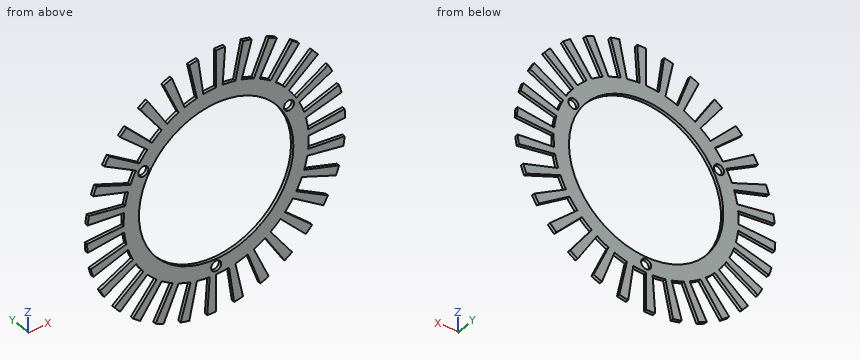
from build123d import *

# Parameters (mm, degrees)
SKETCH1_R           = 30.25
SKETCH1_R_2         = 25.25
EXTRUDE_THIN1_DEPTH = 1
SKETCH2_R           = 1.65
CUT_EXTRUDE3_DEPTH  = 10
BOSS_EXTRUDE1_DEPTH = 1


with BuildPart() as part:
    # Sketch1 → Extrude-Thin1 (new body)
    with BuildSketch(Plane(origin=(0, 0, 0), x_dir=(1, 0, 0), z_dir=(0, 1, 0))):
        Circle(SKETCH1_R)
        Circle(SKETCH1_R_2, mode=Mode.SUBTRACT)
    extrude(amount=-EXTRUDE_THIN1_DEPTH)

    # Sketch2 → Cut-Extrude3 (cut)
    with BuildSketch(Plane(origin=(0, 0, 0), x_dir=(1, 0, 0), z_dir=(0, 1, 0))):
        with Locations((0, 27.5)):
            Circle(SKETCH2_R)
        with Locations((23.815698604, -13.75)):
            Circle(SKETCH2_R)
        with Locations((-23.815698604, -13.75)):
            Circle(SKETCH2_R)
    extrude(amount=-CUT_EXTRUDE3_DEPTH, mode=Mode.SUBTRACT)

    # Sketch5 → Boss-Extrude1 (add)
    with BuildSketch(Plane.XZ.offset(1)):
        with BuildLine():
            Line((0, 42.25), (0, 30.25))
            ThreePointArc((0, 30.25), (1.055709775, 30.231572517), (2.110133331, 30.17631252))
            Line((2.110133331, 30.17631252), (2.947211016, 42.147081123))
            ThreePointArc((2.947211016, 42.147081123), (1.474503736, 42.224262442), (0, 42.25))
        make_face()
        with BuildLine():
            Line((8.784268937, 41.326736131), (6.289328647, 29.588964922))
            ThreePointArc((6.289328647, 29.588964922), (7.318137342, 29.35144572), (8.338030013, 29.078166302))
            Line((8.338030013, 29.078166302), (11.645678283, 40.613306653))
            ThreePointArc((11.645678283, 40.613306653), (10.221200089, 40.994994435), (8.784268937, 41.326736131))
        make_face()
        with BuildLine():
            Line((17.18462317, 38.597295585), (12.303783453, 27.634750094))
            ThreePointArc((12.303783453, 27.634750094), (13.26072719, 27.188519901), (14.201514774, 26.709164684))
            Line((14.201514774, 26.709164684), (19.835173528, 37.304535798))
            ThreePointArc((19.835173528, 37.304535798), (18.521180952, 37.974048456), (17.18462317, 38.597295585))
        make_face()
        with BuildLine():
            Line((24.833926909, 34.180968012), (17.780503882, 24.47276408))
            ThreePointArc((17.780503882, 24.47276408), (18.623759629, 23.837325297), (19.444325193, 23.172844404))
            Line((19.444325193, 23.172844404), (27.157776509, 32.365377722))
            ThreePointArc((27.157776509, 32.365377722), (26.011697333, 33.29345434), (24.833926909, 34.180968012))
        make_face()
        with BuildLine():
            Line((31.397868876, 28.270768119), (22.480130971, 20.241200842))
            ThreePointArc((22.480130971, 20.241200842), (23.172844404, 19.444325193), (23.837325297, 18.623759629))
            Line((23.837325297, 18.623759629), (33.29345434, 26.011697333))
            ThreePointArc((33.29345434, 26.011697333), (32.365377722, 27.157776509), (31.397868876, 28.270768119))
        make_face()
        with BuildLine():
            Line((36.58957331, 21.125), (26.197268464, 15.125))
            ThreePointArc((26.197268464, 15.125), (26.709164684, 14.201514774), (27.188519901, 13.26072719))
            Line((27.188519901, 13.26072719), (37.974048456, 18.521180952))
            ThreePointArc((37.974048456, 18.521180952), (37.304535798, 19.835173528), (36.58957331, 21.125))
        make_face()
        with BuildLine():
            Line((40.182137813, 13.055968012), (28.769459618, 9.34776408))
            ThreePointArc((28.769459618, 9.34776408), (29.078166302, 8.338030013), (29.35144572, 7.318137342))
            Line((29.35144572, 7.318137342), (40.994994435, 10.221200089))
            ThreePointArc((40.994994435, 10.221200089), (40.613306653, 11.645678283), (40.182137813, 13.055968012))
        make_face()
        with BuildLine():
            Line((42.018550079, 4.416327573), (30.084287335, 3.161986014))
            ThreePointArc((30.084287335, 3.161986014), (30.17631252, 2.110133331), (30.231572517, 1.055709775))
            Line((30.231572517, 1.055709775), (42.224262442, 1.474503736))
            ThreePointArc((42.224262442, 1.474503736), (42.147081123, 2.947211016), (42.018550079, 4.416327573))
        make_face()
        with BuildLine():
            Line((42.018550079, -4.416327573), (30.084287335, -3.161986014))
            ThreePointArc((30.084287335, -3.161986014), (29.955609079, -4.209986304), (29.790434529, -5.252857374))
            Line((29.790434529, -5.252857374), (41.608127565, -7.336635506))
            ThreePointArc((41.608127565, -7.336635506), (41.838825904, -5.880063516), (42.018550079, -4.416327573))
        make_face()
        with BuildLine():
            Line((40.182137813, -13.055968012), (28.769459618, -9.34776408))
            ThreePointArc((28.769459618, -9.34776408), (28.425701779, -10.346109336), (28.047311601, -11.331849451))
            Line((28.047311601, -11.331849451), (39.173517855, -15.827128572))
            ThreePointArc((39.173517855, -15.827128572), (39.702013228, -14.450351056), (40.182137813, -13.055968012))
        make_face()
        with BuildLine():
            Line((36.58957331, -21.125), (26.197268464, -15.125))
            ThreePointArc((26.197268464, -15.125), (25.653454909, -16.030057743), (25.07838657, -16.91558533))
            Line((25.07838657, -16.91558533), (35.02683744, -23.625900172))
            ThreePointArc((35.02683744, -23.625900172), (35.830032063, -22.389088914), (36.58957331, -21.125))
        make_face()
        with BuildLine():
            Line((31.397868876, -28.270768119), (22.480130971, -20.241200842))
            ThreePointArc((22.480130971, -20.241200842), (21.76002896, -21.013415706), (21.013415706, -21.76002896))
            Line((21.013415706, -21.76002896), (29.349316152, -30.392106564))
            ThreePointArc((29.349316152, -30.392106564), (30.392106564, -29.349316152), (31.397868876, -28.270768119))
        make_face()
        with BuildLine():
            Line((24.833926909, -34.180968012), (17.780503882, -24.47276408))
            ThreePointArc((17.780503882, -24.47276408), (16.91558533, -25.07838657), (16.030057743, -25.653454909))
            Line((16.030057743, -25.653454909), (22.389088914, -35.830032063))
            ThreePointArc((22.389088914, -35.830032063), (23.625900172, -35.02683744), (24.833926909, -34.180968012))
        make_face()
        with BuildLine():
            Line((17.18462317, -38.597295585), (12.303783453, -27.634750094))
            ThreePointArc((12.303783453, -27.634750094), (11.331849451, -28.047311601), (10.346109336, -28.425701779))
            Line((10.346109336, -28.425701779), (14.450351056, -39.702013228))
            ThreePointArc((14.450351056, -39.702013228), (15.827128572, -39.173517855), (17.18462317, -38.597295585))
        make_face()
        with BuildLine():
            Line((8.784268937, -41.326736131), (6.289328647, -29.588964922))
            ThreePointArc((6.289328647, -29.588964922), (5.252857374, -29.790434529), (4.209986304, -29.955609079))
            Line((4.209986304, -29.955609079), (5.880063516, -41.838825904))
            ThreePointArc((5.880063516, -41.838825904), (7.336635506, -41.608127565), (8.784268937, -41.326736131))
        make_face()
        with BuildLine():
            Line((0, -42.25), (0, -30.25))
            ThreePointArc((0, -30.25), (-1.055709775, -30.231572517), (-2.110133331, -30.17631252))
            Line((-2.110133331, -30.17631252), (-2.947211016, -42.147081123))
            ThreePointArc((-2.947211016, -42.147081123), (-1.474503736, -42.224262442), (0, -42.25))
        make_face()
        with BuildLine():
            Line((-8.784268937, -41.326736131), (-6.289328647, -29.588964922))
            ThreePointArc((-6.289328647, -29.588964922), (-7.318137342, -29.35144572), (-8.338030013, -29.078166302))
            Line((-8.338030013, -29.078166302), (-11.645678283, -40.613306653))
            ThreePointArc((-11.645678283, -40.613306653), (-10.221200089, -40.994994435), (-8.784268937, -41.326736131))
        make_face()
        with BuildLine():
            Line((-17.18462317, -38.597295585), (-12.303783453, -27.634750094))
            ThreePointArc((-12.303783453, -27.634750094), (-13.26072719, -27.188519901), (-14.201514774, -26.709164684))
            Line((-14.201514774, -26.709164684), (-19.835173528, -37.304535798))
            ThreePointArc((-19.835173528, -37.304535798), (-18.521180952, -37.974048456), (-17.18462317, -38.597295585))
        make_face()
        with BuildLine():
            Line((-24.833926909, -34.180968012), (-17.780503882, -24.47276408))
            ThreePointArc((-17.780503882, -24.47276408), (-18.623759629, -23.837325297), (-19.444325193, -23.172844404))
            Line((-19.444325193, -23.172844404), (-27.157776509, -32.365377722))
            ThreePointArc((-27.157776509, -32.365377722), (-26.011697333, -33.29345434), (-24.833926909, -34.180968012))
        make_face()
        with BuildLine():
            Line((-31.397868876, -28.270768119), (-22.480130971, -20.241200842))
            ThreePointArc((-22.480130971, -20.241200842), (-23.172844404, -19.444325193), (-23.837325297, -18.623759629))
            Line((-23.837325297, -18.623759629), (-33.29345434, -26.011697333))
            ThreePointArc((-33.29345434, -26.011697333), (-32.365377722, -27.157776509), (-31.397868876, -28.270768119))
        make_face()
        with BuildLine():
            Line((-36.58957331, -21.125), (-26.197268464, -15.125))
            ThreePointArc((-26.197268464, -15.125), (-26.709164684, -14.201514774), (-27.188519901, -13.26072719))
            Line((-27.188519901, -13.26072719), (-37.974048456, -18.521180952))
            ThreePointArc((-37.974048456, -18.521180952), (-37.304535798, -19.835173528), (-36.58957331, -21.125))
        make_face()
        with BuildLine():
            Line((-40.182137813, -13.055968012), (-28.769459618, -9.34776408))
            ThreePointArc((-28.769459618, -9.34776408), (-29.078166302, -8.338030013), (-29.35144572, -7.318137342))
            Line((-29.35144572, -7.318137342), (-40.994994435, -10.221200089))
            ThreePointArc((-40.994994435, -10.221200089), (-40.613306653, -11.645678283), (-40.182137813, -13.055968012))
        make_face()
        with BuildLine():
            Line((-42.018550079, -4.416327573), (-30.084287335, -3.161986014))
            ThreePointArc((-30.084287335, -3.161986014), (-30.17631252, -2.110133331), (-30.231572517, -1.055709775))
            Line((-30.231572517, -1.055709775), (-42.224262442, -1.474503736))
            ThreePointArc((-42.224262442, -1.474503736), (-42.147081123, -2.947211016), (-42.018550079, -4.416327573))
        make_face()
        with BuildLine():
            Line((-42.018550079, 4.416327573), (-30.084287335, 3.161986014))
            ThreePointArc((-30.084287335, 3.161986014), (-29.955609079, 4.209986304), (-29.790434529, 5.252857374))
            Line((-29.790434529, 5.252857374), (-41.608127565, 7.336635506))
            ThreePointArc((-41.608127565, 7.336635506), (-41.838825904, 5.880063516), (-42.018550079, 4.416327573))
        make_face()
        with BuildLine():
            Line((-40.182137813, 13.055968012), (-28.769459618, 9.34776408))
            ThreePointArc((-28.769459618, 9.34776408), (-28.425701779, 10.346109336), (-28.047311601, 11.331849451))
            Line((-28.047311601, 11.331849451), (-39.173517855, 15.827128572))
            ThreePointArc((-39.173517855, 15.827128572), (-39.702013228, 14.450351056), (-40.182137813, 13.055968012))
        make_face()
        with BuildLine():
            Line((-36.58957331, 21.125), (-26.197268464, 15.125))
            ThreePointArc((-26.197268464, 15.125), (-25.653454909, 16.030057743), (-25.07838657, 16.91558533))
            Line((-25.07838657, 16.91558533), (-35.02683744, 23.625900172))
            ThreePointArc((-35.02683744, 23.625900172), (-35.830032063, 22.389088914), (-36.58957331, 21.125))
        make_face()
        with BuildLine():
            Line((-31.397868876, 28.270768119), (-22.480130971, 20.241200842))
            ThreePointArc((-22.480130971, 20.241200842), (-21.76002896, 21.013415706), (-21.013415706, 21.76002896))
            Line((-21.013415706, 21.76002896), (-29.349316152, 30.392106564))
            ThreePointArc((-29.349316152, 30.392106564), (-30.392106564, 29.349316152), (-31.397868876, 28.270768119))
        make_face()
        with BuildLine():
            Line((-24.833926909, 34.180968012), (-17.780503882, 24.47276408))
            ThreePointArc((-17.780503882, 24.47276408), (-16.91558533, 25.07838657), (-16.030057743, 25.653454909))
            Line((-16.030057743, 25.653454909), (-22.389088914, 35.830032063))
            ThreePointArc((-22.389088914, 35.830032063), (-23.625900172, 35.02683744), (-24.833926909, 34.180968012))
        make_face()
        with BuildLine():
            Line((-17.18462317, 38.597295585), (-12.303783453, 27.634750094))
            ThreePointArc((-12.303783453, 27.634750094), (-11.331849451, 28.047311601), (-10.346109336, 28.425701779))
            Line((-10.346109336, 28.425701779), (-14.450351056, 39.702013228))
            ThreePointArc((-14.450351056, 39.702013228), (-15.827128572, 39.173517855), (-17.18462317, 38.597295585))
        make_face()
        with BuildLine():
            Line((-8.784268937, 41.326736131), (-6.289328647, 29.588964922))
            ThreePointArc((-6.289328647, 29.588964922), (-5.252857374, 29.790434529), (-4.209986304, 29.955609079))
            Line((-4.209986304, 29.955609079), (-5.880063516, 41.838825904))
            ThreePointArc((-5.880063516, 41.838825904), (-7.336635506, 41.608127565), (-8.784268937, 41.326736131))
        make_face()
    extrude(amount=-BOSS_EXTRUDE1_DEPTH)


solid = part.part
Geometry: final body of the model. Coordinates: model frame, mm. Round coordinates to 2 decimals unless told otherwise and drop trailing zeros. Loops run counter-clockwise (first coordinate to the right, second up) from the corner with the lowest first, then second, coordinate; pieces in that order, holes last. Notation, with made-up numbers: M 28.25,5.5 L 60.25,5.5 A9 cw 60.25,11.5 Z; hole C 63.5,18.25 d2. An arc over 180 degrees is marked long. One line per question, with ' | ' between items.
(1) Material intervals for line 1 along X through (y, z) = (-0.55, 25.5); line 2 along X through (y, z) = (-0.6, -16.5); line 3 along X through (y, z) = (-0.6, 13.75), sorted ascending. Write a range as from..to.
Check result:
line 1: x = -28.32..-24.63, -18.53..16.27, 18.53..21.4, 28.32..32.64 | line 2: x = -33.83..-28.58, -25.35..-19.11, 19.11..28.58 | line 3: x = -39.95..-34.03, -26.94..-25.47, -22.17..-21.18, 21.18..22.17, 25.47..28.19
(2) Cut plane B-B on y = -0.5. Give the number of separate pieces and of enclosed holes in the cut face, plus the area to 3 significant figures.
Check result:
separate pieces: 1 | enclosed holes: 4 | area: 1,760 mm2
(3) Cut plane A-A on z = 0. Return the cut outline in (x, y).
Check result:
outline: M -30.25,-1 L -25.25,-1 L -25.25,0 L -30.25,0 Z; M 25.25,-1 L 30.25,-1 L 30.25,0 L 25.25,0 Z
(4) Contact query for a flat-ended pin moving along its axis: P1, Ø3, axis at x = -23.82, z = 13.75, coming from the +Y side. Output: stop coordinate, or through.
Check result:
P1: passes through
